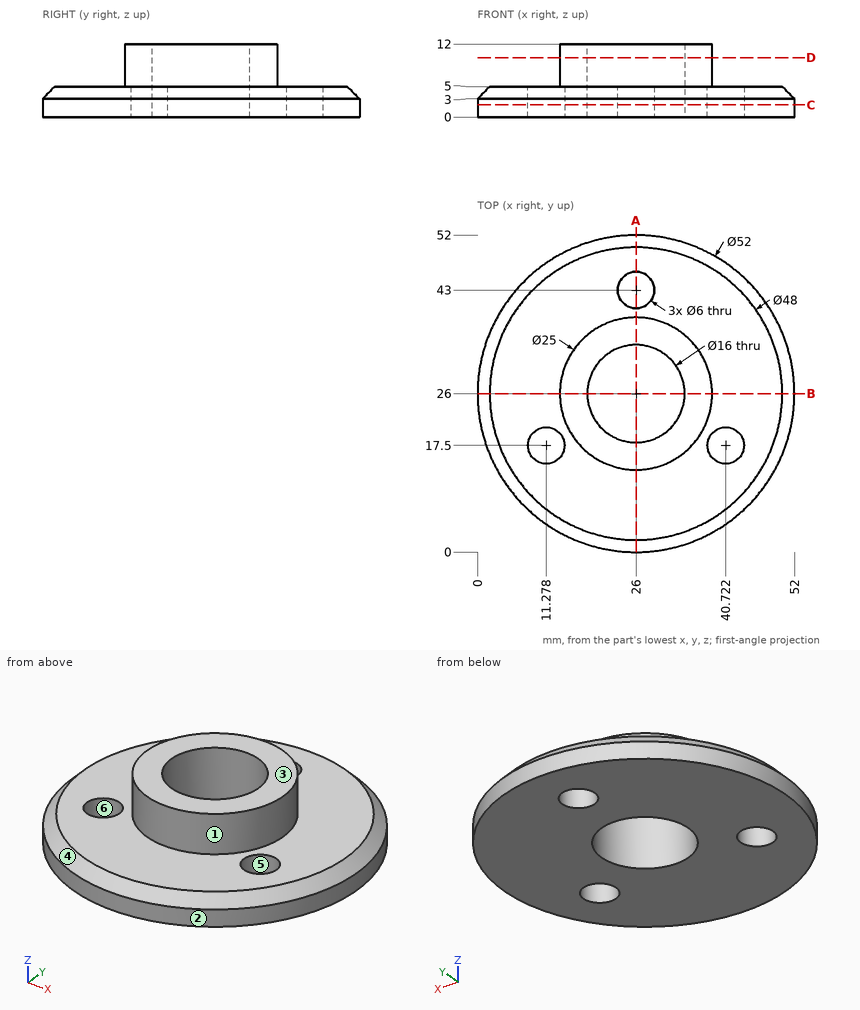
Geometry check sheet. Reference: drawing and pictorial views, mm from the part's lowest x, y, z. A direction names the side the tool comes from. Give positions to 0.01 mm unless a question says otherwise; leave off trailing zeros. Write each loop counter-clockwise with the first axis right and the second up, starting at its lowest first coordinate (ties: lowest second). Pieces come first, ordered by that corner, then holes. Notation, with made-up numbers: (-21, -4.5) -> (18, -4.5) arc R10 cw to (18, 10.5) -> close; hole circle Ø11 at (-31.5, 34). An arc over 180 degrees is marked (long way). One line per question, with ' | ' between items.
Item 1: Depth check by flat-ended pin: pin 1 (6 mm diameter, centred on x = 42.5, z = 4.5, fed in from +Y); pin 2 (4 mm diameter, centred on x = 28, y = 43.5, fed in from +Z); pin 3 (10 mm diameter, centred on x = 18.5, y = 18.5, fed in from -Z). Enter the tip coordinate at first touch or a pass-through.
Determined:
pin 1: y = 47.97 | pin 2: z = 5 | pin 3: z = 0
Item 2: Access from +Z, -Z, +X, -X, +Y, -Y to the whole of each face (thin tool, end or side, straight path). Record for the marked faces 1 and 2.
Determined:
face 1: +Z | face 2: +Z, -Z
Item 3: Sectioned sample at B-B, the plane y = 26. Record the boundary of the cut face in (x, z).
Determined:
outline: (0, 0) -> (18, 0) -> (18, 12) -> (13.5, 12) -> (13.5, 5) -> (2, 5) -> (0, 3) -> close; (34, 0) -> (52, 0) -> (52, 3) -> (50, 5) -> (38.5, 5) -> (38.5, 12) -> (34, 12) -> close
Item 4: Sectioned sample at A-A, the plane x = 26. Record the boundary of the cut face in (y, z).
Determined:
outline: (0, 0) -> (18, 0) -> (18, 12) -> (13.5, 12) -> (13.5, 5) -> (2, 5) -> (0, 3) -> close; (34, 0) -> (40, 0) -> (40, 5) -> (38.5, 5) -> (38.5, 12) -> (34, 12) -> close; (46, 0) -> (52, 0) -> (52, 3) -> (50, 5) -> (46, 5) -> close
Item 5: Draft check along X on the marked faces 3, 4, 5 and 6. Enter one of: released by +X, released by -X, zero draft, split by the parting line, or undercut.
Determined:
face 3: zero draft | face 4: split by the parting line | face 5: undercut | face 6: undercut
Item 6: Sectioned sample at D-D, the plane z = 9.75. Record the boundary of the cut face in (x, y), plus the area to 3 significant figures.
Determined:
outline: circle Ø25 at (26, 26); hole circle Ø16 at (26, 26) | area: 290 mm^2
Item 7: Sectioned sample at C-C, the plane z = 2. Record the boundary of the cut face in (x, y).
Determined:
outline: circle Ø52 at (26, 26); hole circle Ø6 at (11.28, 17.5); hole circle Ø16 at (26, 26); hole circle Ø6 at (26, 43); hole circle Ø6 at (40.72, 17.5)
Item 8: Scan lines: line 1 along Y through (x, z) = (26, 1.1); line 2 along Y through (x, z) = (26, 8); line 3 along Y through (x, z) = (26, 3.5). Record each from-to range of solid material in increasing order.
Determined:
line 1: 0 to 18, 34 to 40, 46 to 52 | line 2: 13.5 to 18, 34 to 38.5 | line 3: 0.5 to 18, 34 to 40, 46 to 51.5
